Geometry: final body of the model. Coordinates: model frame, mm. A direction names the side the tool comes from. Round coordinates to 2 decimals unless told otherwise and drop trailing zeros. Loops run counter-clockwise (first coordinate to the right, second up) from the corner with the lowest first, then second, coordinate; pieces in that order, holes last. Notation, with made-up numbers: (78.5, 64.5) - (128.5, 64.5) arc R21 ccw to (128.5, 89.5) - close; hole circle Ø2 at (37, 10.5). An arc over 180 degrees is marked (long way). Answer as CSV lines item,"result".
Autodesk Inventor part; units mm, degrees
ref_plane "Work Plane1" through (0, 0, 0) normal (0, 0, 1) x (1, 0, 0)
ref_plane "YZ Plane" through (0, 0, 0) normal (1, 0, 0) x (0, 1, 0)
ref_plane "XZ Plane" through (0, 0, 0) normal (0, 1, 0) x (-1, 0, 0)
ref_plane "Work Plane1" through (0, 0, 0) normal (0, 0, 1) x (1, 0, 0)
sketch "Sketch1" plane through (0, 0, 0) normal (0, 0, 1) x (1, 0, 0)
  line L0 (195.6597, 725) -> (745.6597, 725)
  line L1 (745.6597, 725) -> (745.6597, 775)
  line L2 (745.6597, 775) -> (195.6597, 775)
  line L3 (195.6597, 775) -> (195.6597, 725)
  line L4 (164.0316, 10) -> (164.0316, 1490)
  line L5 (777.2877, 10) -> (164.0316, 10)
  line L6 (470.6597, 10) -> (470.6597, 1506) construction
  line L7 (164.0316, 750) -> (680, 750) construction
  point P0 (0, 0)
  point P1 (470.6597, 725)
  point P2 (195.6597, 750)
  dimension "d0" = 550
  dimension "d1" = 50
extrude "Extrusion1" add sketch "Sketch1" along normal blind 15
sketch "Sketch2" plane through (195.6597, 725, 0) normal (-1, 0, 0) x (0, 0, 1)
  line L0 (15, 0) -> (0, 0)
  line L1 (0, 0) -> (0, 50)
  line L2 (0, 50) -> (15, 50)
  line L3 (15, 50) -> (15, 0)
  line L4 (12, 48) -> (0, 48)
  line L5 (0, 2) -> (12, 2)
  line L6 (13, 3) -> (13, 47)
  arc A0 (13, 47) -> (12, 48) centre (12, 47) ccw
  arc A1 (12, 2) -> (13, 3) centre (12, 3) ccw
  point P0 (0, -725)
  dimension "d5" = 2
extrude "Extrusion2" cut sketch "Sketch2" against normal through all contours L1 L4 A0 L6 A1 L5
fillet "Fillet1" radius 2 4 edges at (470.6597, 775, 15) (470.6597, 775, 0) (470.6597, 725, 0) (470.6597, 725, 15)
sketch "Sketch3" plane through (0, 0, 15) normal (0, 0, 1) x (1, 0, 0)
  line L0 (195.6597, 727) -> (745.6597, 727) construction
  line L1 (745.6597, 773) -> (745.6597, 727) construction
  line L2 (745.6597, 773) -> (195.6597, 773) construction
  line L3 (195.6597, 727) -> (195.6597, 773) construction
  line L4 (195.6597, 772) -> (745.6597, 772)
  line L5 (470.6597, 772) -> (470.6597, 727) construction
  circle A0 centre (470.6597, 749.5) radius 5
  point P0 (0, 0)
  dimension "d10" = 10
extrude "Extrusion3" cut sketch "Sketch3" against normal up to next
pattern_linear "Rectangular Pattern1" count 5 spacing 120 along (1, 0, 0) of "Extrusion3" first direction both ways yes
properties part number "support1" material "Stainless Steel"
(1) Access query for faces 1 (the face through (467, 773, 6)), 2 (the face through (467, 755, 15)). Directions: +Z, -Z, +X, -X, +Y, -Y. A direction counts if a zero-diameter tool reaches every point of the face in a straight line with its end or side. Return the directions, or none.
Findings below:
face 1,"-Z, +X, -X"
face 2,"+Z, +X, -X, +Y, -Y"
(2) Pin query (flat end, axial travel): P1, Ø16, axis at x = 590.66, y = 749.5, coming from the -Z side. Return the tip coordinate at first contact, or that it passes through.
Findings below:
P1,"z = 13"
(3) Section A-A (z = 6). Output: boundary loops of the cut face in (x, y), and give its area (3 significant figures).
Findings below:
outline,"(195.66, 725) - (745.66, 725) - (745.66, 727) - (195.66, 727) - close; (195.66, 773) - (745.66, 773) - (745.66, 775) - (195.66, 775) - close"
area,"2,200 mm2"
(4) Section B-B (y = 749.5). Output: boundary loops of the cut face in (x, z), and give its area (3 significant figures).
Findings below:
outline,"(195.66, 13) - (225.66, 13) - (225.66, 15) - (195.66, 15) - close; (235.66, 13) - (345.66, 13) - (345.66, 15) - (235.66, 15) - close; (355.66, 13) - (465.66, 13) - (465.66, 15) - (355.66, 15) - close; (475.66, 13) - (585.66, 13) - (585.66, 15) - (475.66, 15) - close; (595.66, 13) - (705.66, 13) - (705.66, 15) - (595.66, 15) - close; (715.66, 13) - (745.66, 13) - (745.66, 15) - (715.66, 15) - close"
area,"1,000 mm2"
(5) Draft query along X for faces 3 (the face through (195.66, 750, 14)), 4 (the face through (745.66, 750, 14)), 5 (the face through (229.58, 744.62, 14.01)), 6 (the face through (475, 775, 7)). Return one class per face: pulls with the +X half, pulls with the -X half, needs draft (parallel to the pull), parting line crosses it, or undercut.
Findings below:
face 3,"pulls with the -X half"
face 4,"pulls with the +X half"
face 5,"undercut"
face 6,"needs draft"
(6) Material intervals for line 1 along X through (y, z) = (749.5, 14.05); line 2 along Y through (x, z) = (608.5, 8.25); line 3 along Z through (x, y) = (610.5, 738), sorted ascending.
Findings below:
line 1,"195.66 to 225.66, 235.66 to 345.66, 355.66 to 465.66, 475.66 to 585.66, 595.66 to 705.66, 715.66 to 745.66"
line 2,"725 to 727, 773 to 775"
line 3,"13 to 15"
